The listing builds one solid part. Answer for the finished solid, in the listing's coordinates (mm). Give positions to 0.01 mm unless a question says otherwise; leave off trailing zeros. Order: outer loops, then holes, each group sorted by start corner. A loop starts at its lowest first (then second) coordinate and runs counter-clockwise, first axis right, second up. Notation, with made-up numbers: (76.25, 73.25) - (133.25, 73.25) arc R9 ccw to (133.25, 79.25) - close; hole circle Ø10 at (1.5, 61.25). An arc over 180 degrees is marked (long way). Answer in a Markdown table with one row per item.
from build123d import *

# Parameters (mm, degrees)
BOSS_EXTRUDE1_DEPTH = 38.1


with BuildPart() as part:
    # Sketch1 → Boss-Extrude1 (new body, symmetric)
    with BuildSketch(Plane.XY):
        with BuildLine():
            Line((487.3625, 481.378335213), (487.3625, 359.522344396))
            Line((487.3625, 359.522344396), (481.0125, 359.522344396))
            ThreePointArc((481.0125, 359.522344396), (474.121977685, 386.119365688), (464.802007403, 411.965429089))
            ThreePointArc((464.802007403, 411.965429089), (462.872580153, 421.889683903), (464.967167576, 431.780398065))
            ThreePointArc((464.967167576, 431.780398065), (474.183122715, 456.193328053), (481.0125, 481.378335213))
            Line((481.0125, 481.378335213), (487.3625, 481.378335213))
        make_face()
    extrude(amount=BOSS_EXTRUDE1_DEPTH, both=True)


solid = part.part
Item 1: Find section B-B on y = 447.5. Write down the section's boundary in (x, z), then the cut area to 3 significant figures.
Answer block:
| item | result |
|---|---|
| outline | (471.21, -38.1) - (487.36, -38.1) - (487.36, 38.1) - (471.21, 38.1) - close |
| area | 1,230 mm² |
Item 2: Each of these flat-tipped pins is pushed along its axis until it touches: P1, Ø10, axis at x = 474.5, y = 384, coming from the -Z side; P2, Ø1, axis at y = 406, z = 8, coming from the -X side; P3, Ø12, axis at y = 376, z = 4, coming from the -X side. Where does it stop, or does it pass through?
Answer block:
| item | result |
|---|---|
| P1 | z = -38.1 |
| P2 | x = 467 |
| P3 | x = 475.36 |
Item 3: Consider line 1 (X direction, y = 476, z = -15); line 2 (X direction, y = 402, z = -9.5); line 3 (Y direction, x = 466.25, z = 29). Determine where each line is inside the solid, lowest interval first.
Answer block:
| item | result |
|---|---|
| line 1 | 479.77 to 487.36 |
| line 2 | 468.72 to 487.36 |
| line 3 | 408.4 to 434.79 |
Item 4: Find section C-C on x = 468. Write down the section's boundary in (y, z).
Answer block:
| item | result |
|---|---|
| outline | (403.91, -38.1) - (439.06, -38.1) - (439.06, 38.1) - (403.91, 38.1) - close |
